```python
from build123d import *

# Parameters (mm, degrees)
F0_R     = 11
F0_R_2   = 5.5
F0_R_3   = 4.1
F1_DEPTH = 3
F2_DEPTH = 4.25
F3_SIZE  = 0.7
F4_R     = 0.9
F5_DEPTH = 0.5
F7_DEPTH = 0.5


with BuildPart() as f1:
    # F0 (on Top) → F1 (new body)
    with BuildSketch(Plane.XY):
        Circle(F0_R)
        Circle(F0_R_2, mode=Mode.SUBTRACT)
        Circle(F0_R_2)
        Circle(F0_R_3, mode=Mode.SUBTRACT)
        Circle(F0_R_3)
    extrude(amount=F1_DEPTH)

    # F0 (on Top) → F2 (join)
    with BuildSketch(Plane.XY):
        Circle(F0_R_3)
    extrude(amount=-F2_DEPTH)

    # F3
    f3_edges = [f1.edges().sort_by_distance(p)[0] for p in [
        (-4.1, 0, -4.25),
    ]]
    chamfer(f3_edges, length=F3_SIZE)

    # F4
    f4_edges = [f1.edges().sort_by_distance(p)[0] for p in [
        (11, 0, 1.5),
        (-11, 0, 0),
        (-11, 0, 3),
    ]]
    fillet(f4_edges, radius=F4_R)

    # F0 (on Top) → F5 (join)
    with BuildSketch(Plane.XY):
        Circle(F0_R_2)
        Circle(F0_R_3, mode=Mode.SUBTRACT)
    extrude(amount=-F5_DEPTH)

    # F6 (on face) → F7 (cut)
    with BuildSketch(Plane.XY.offset(3)):
        with BuildLine():
            ThreePointArc((1.3453624047, -9), (3.7170414054, -8.3062388113), (5.814636704, -7))
            Line((5.814636704, -7), (-5.814636704, -7))
            ThreePointArc((-5.814636704, -7), (-3.7170414054, -8.3062388113), (-1.3453624047, -9))
            Line((-1.3453624047, -9), (1.3453624047, -9))
        make_face()
        with BuildLine():
            ThreePointArc((7.6032887621, -5), (8.1587971524, -4.0303881979), (8.5912746435, -3))
            Line((8.5912746435, -3), (-8.5912746435, -3))
            ThreePointArc((-8.5912746435, -3), (-8.1587971524, -4.0303881979), (-7.6032887621, -5))
            Line((-7.6032887621, -5), (7.6032887621, -5))
        make_face()
        with BuildLine():
            ThreePointArc((9.044888059, -1), (9.0862115686, -0.5007587558), (9.1, 0))
            ThreePointArc((9.1, 0), (9.0862115686, 0.5007587558), (9.044888059, 1))
            Line((9.044888059, 1), (-9.044888059, 1))
            ThreePointArc((-9.044888059, 1), (-9.1, 0), (-9.044888059, -1))
            Line((-9.044888059, -1), (9.044888059, -1))
        make_face()
        with BuildLine():
            Line((-8.5912746435, 3), (8.5912746435, 3))
            ThreePointArc((8.5912746435, 3), (8.1587971524, 4.0303881979), (7.6032887621, 5))
            Line((7.6032887621, 5), (-7.6032887621, 5))
            ThreePointArc((-7.6032887621, 5), (-8.1587971524, 4.0303881979), (-8.5912746435, 3))
        make_face()
        with BuildLine():
            Line((-5.814636704, 7), (5.814636704, 7))
            ThreePointArc((5.814636704, 7), (3.7170414054, 8.3062388113), (1.3453624047, 9))
            Line((1.3453624047, 9), (-1.3453624047, 9))
            ThreePointArc((-1.3453624047, 9), (-3.7170414054, 8.3062388113), (-5.814636704, 7))
        make_face()
        with BuildLine():
            ThreePointArc((-1.3453624047, -9), (0, -9.1), (1.3453624047, -9))
            Line((1.3453624047, -9), (-1.3453624047, -9))
        make_face()
        with BuildLine():
            Line((-1.3453624047, 9), (1.3453624047, 9))
            ThreePointArc((1.3453624047, 9), (0, 9.1), (-1.3453624047, 9))
        make_face()
    extrude(amount=-F7_DEPTH, mode=Mode.SUBTRACT)


solid = f1.part
```
Can you work these out from the model? Positions are in its coordinate system, mm. A direction names the side the tool comes from. Round coordinates to 2 decimals unless told otherwise and drop trailing zeros. Loops run counter-clockwise (first coordinate to the right, second up) from the corner with the lowest first, then second, coordinate; pieces in that order, holes last. Notation, with made-up numbers: (11.25, 9) -> (46.25, 9) arc R14 ccw to (46.25, 21) -> close; hole circle Ø9 at (35, 77.25). An arc over 180 degrees is marked (long way). One line per item, written item: value. Start each with the question number.
1. For pin 1 (5 mm diameter, centred on x = 5.5, y = -7, fed in from -Z); pin 2 (4 mm diameter, centred on x = -3, z = -1, fed in from -Y); pin 3 (8 mm diameter, centred on x = -8, y = 2, fed in from -Z), each with a flat end and sliding along its axis, tell me the tip position at first contact or that it passes through.
2. If I drill on probe 1 along Y at (x, z) = (-1.75, 2.75); probe 2 along Z at (x, y) = (6.75, 0); probe 3 along Z at (x, y) = (-9.25, 4.25), over which ranges is the centre line in solid material (lowest first)?
3. If we mould it in two halves opening along Y, with no side actions, what happens to faces 4 (the cylindrical face through (-1.19, -5.37, -0.25)), 5 (the flat face through (0, 4, 2.5)), 6 (the flat face through (0, 2, 3))? For each: pulls with the +Y half, pulls with the -Y half, needs draft (parallel to the pull), parting line crosses it, or undercut.
4. If we section it at A-A, the plane z = -1.5: Write out the boundary of the cut face in (x, y).
5. If we section it at B-B, the plane z = 1.75: Write out the boundary of the cut face in (x, y), then the cut area to 3 significant figures.
6. For faces 1 (the cylindrical face through (-2.38, -10.74, 1.49)), 2 (the flat face through (4, -4, 0)), 3 (the flat face through (0, 8, 2.5)), which set-ups out of +Z, -Z, +X, -X, +Y, -Y let a thin tool reach every point of the face, with its end or its side?
Calculated:
1. pin 1: stops at z = 0
1. pin 2: stops at y = -10.8
1. pin 3: stops at z = -0.5
2. probe 1: y = -10.58 to -8.93, -7 to -5, -3 to -1, 1 to 3, 5 to 7, 8.93 to 10.58
2. probe 2: z = 0 to 2.5
2. probe 3: z = 0 to 3
3. face 4: parting line crosses it
3. face 5: undercut
3. face 6: needs draft
4. outline: circle Ø8.2 at (0, 0)
5. outline: circle Ø22 at (0, 0)
5. area: 380 mm²
6. face 1: +Z, -Z
6. face 2: -Z
6. face 3: +Z
